Autodesk Inventor part; units mm, degrees
ref_plane "Work Plane1" through (0, -35, 0) normal (0, 1, 0) x (-1, 0, 0)
ref_plane "YZ Plane" through (0, 0, 0) normal (1, 0, 0) x (0, 1, 0)
ref_plane "XY Plane" through (0, 0, 0) normal (0, 0, 1) x (1, 0, 0)
sketch "Sketch1" plane through (0, 0, 0) normal (0, 0, 1) x (1, 0, 0)
  circle A0 centre (0, 0) radius 25
  circle A1 centre (0, 0) radius 35
  line L0 (-17.6777, 17.6777) -> (-24.7487, 24.7487)
  line L1 (0, 35) -> (0, 0) construction
  line L2 (-24.0315, 25.4457) -> (-16.9564, 18.3706)
  line L3 (-1.1667, 34.9806) -> (-1.1667, 34.9972)
  line L4 (1.1667, 34.9806) -> (1.1667, 34.9972)
  line L5 (17.6777, 17.6777) -> (24.7487, 24.7487)
  line L6 (24.0315, 25.4457) -> (16.9564, 18.3706)
  line L7 (-25.4457, 24.0315) -> (-18.3706, 16.9564)
  line L8 (25.4457, 24.0315) -> (18.3706, 16.9564)
  line L9 (-1, 15) -> (1, 15)
  line L10 (1, 15) -> (1, 0)
  line L11 (1, 0) -> (-1, 0)
  line L12 (-1, 0) -> (-1, 15)
  line L13 (-1, 0) -> (1, 0)
  line L14 (1, 0) -> (1, -7)
  line L15 (1, -7) -> (-1, -7)
  line L16 (-1, -7) -> (-1, 0)
  line L17 (-1, -7) -> (-5, -7)
  line L18 (-5, -7) -> (-5, 4)
  line L19 (-5, 4) -> (-1, 4)
  line L20 (-1, 4) -> (-1, -7)
  line L21 (-5, 4) -> (-21.5953, -12.5953)
  line L22 (-5, -7) -> (-16.6494, -18.6494)
  line L23 (-5, 4) -> (-1, 15)
  line L24 (-5, -7) -> (-1, -3)
  line L25 (1, 0) -> (1, 15)
  line L26 (1, -7) -> (1, 0)
  line L27 (5, 4) -> (21.5953, -12.5953)
  line L28 (5, -7) -> (16.6494, -18.6494)
  line L29 (5, 4) -> (1, 15)
  line L30 (5, -7) -> (1, -3)
  point P0 (-20.5061, 21.9203)
  point P1 (-21.9203, 20.5061)
  point P2 (20.5061, 21.9203)
  point P3 (21.9203, 20.5061)
  point P4 (-1, -3)
  point P5 (1, 0)
  point P6 (1, -3)
  point P7 (21.5953, -12.5953)
  dimension "d0" = 50
  dimension "d1" = 10
  dimension "d2" = 45
  dimension "d3" = 1
  dimension "d5" = 2
  dimension "d6" = 15
  dimension "d7" = 7
  dimension "d8" = 2
  dimension "d9" = 4
  dimension "d11" = 45
  dimension "d12" = 45
  dimension "d13" = 4
  dimension "d14" = 45
extrude "Extrusion1" add sketch "Sketch1" along normal blind 10 contours A0 L8 A1 L7 | A0 L28 L30 L14 L10 L29 L27 | A0 L21 L18 L22 | L18 L19 L12 L16 L24 | L12 L19 L23
sketch "Sketch2" plane through (0, 0, 0) normal (0, 0, 1) x (1, 0, 0)
  point P0 (0, 0)
extrude "Extrusion2" add sketch "Sketch1" along normal blind 5 contours A0 L5 A1 L8 | A0 L6 A1 L5 | A0 L2 A1 L6 | A0 L0 A1 L2 | A1 L0 A0 L7
sketch "Sketch4" plane through (0, 0, 5) normal (0, 0, 1) x (1, 0, 0)
  arc A0 (18.3706, 16.9564) -> (-18.3706, 16.9564) centre (0, 0) ccw construction
  circle A1 centre (0, 30) radius 2.5
  point P0 (0, 25)
  dimension "d19" = 5
  dimension "d20" = 5
extrude "Extrusion3" cut sketch "Sketch4" against normal through all
chamfer "Chamfer1" distance 1 angle 45 1 edges at (-2.5, 30, 5)
ref_plane "Work Plane1" through (0, -35, 0) normal (0, 1, 0) x (-1, 0, 0)
sketch "Sketch6" plane through (0, -35, 0) normal (0, 1, 0) x (-1, 0, 0)
  line L0 (3.5, 5) -> (-3.5, 5) construction
  circle A0 centre (0, 5) radius 4.9
  point P0 (0, 0)
  dimension "d27" = 9.8
extrude "Extrusion4" add sketch "Sketch6" along normal blind 5 and the other way blind 20
chamfer "Chamfer2" distance 1 angle 45 1 edges at (4.9, -55, 5)
properties part number "Black_Part1"
Verification items for the finished model (mm, model axes). A direction names the side the tool comes from. Round coordinates to 2 decimals unless told otherwise and drop trailing zeros. Order: outer loops, then holes, each group sorted by start corner. A loop starts at its lowest first (then second) coordinate and runs counter-clockwise, first axis right, second up. Notation, with made-up numbers: (9, 5.5) -> (68, 5.5) arc R23 ccw to (68, 13.5) -> close; hole circle Ø5 at (20.25, 45.25). An arc over 180 degrees is marked (long way). Put each result on its own line as item: value. Start each with the question number.
(1) Section check A-A (y = 0). Enter the section's corners in (x, z).
(2) Draft check along Y on faces 1 (the face through (3.03, 9.42, 4.93)), 2 (the face through (21.958, 20.543, 7.465)), 3 (the face through (0, 26, 5)). Enter one of: +Y half, -Y half, draft (parallel to the pull), parting line (faces both ways), or undercut.
(3) Material ranges on line 1 along Y through (x, z) = (0, 1.35); line 2 along Y through (x, z) = (9, 0.5); line 3 along X through (y, z) = (0, 3.5), recorded low to high.
(4) Section check D-D (y = -44.5). Enter the section's corners in (x, z), then the cut area to 3 significant figures.
(5) Section check B-B (y = 30). Enter the section's corners in (x, z), then the cut area to 3 significant figures.
(6) Depth check by flat-ended pin: pin 1 Ø6 at (y, z) = (-24, 8.5) entering from -X; pin 2 Ø1.5 at (y, z) = (-11, 9) entering from -X; pin 3 Ø1.5 at (x, z) = (26.5, 1.5) entering from -Y. Enter the tip coordinate at first touch or a pass-through.
(7) Section check C-C (x = -8.5). Enter the section's corners in (y, z).
(8) Tool access check on faces 4 (the face through (0, -25, 5)), 5 (the face through (-21.958, 20.543, 7.465)), 6 (the face through (0, -55, 5)), 7 (the face through (1.062, -44.463, 9.783)), 8 (the face through (7, 0, 0)). Record the directions out of +Z, -Z, +X, -X, +Y, -Y that give a thin tool (end or side, any length) a straight path to the whole face; none if there is none.
Completed:
1. outline: (-35, 0) -> (-25, 0) -> (-25, 10) -> (-35, 10) -> close; (-9, 0) -> (-1, 0) -> (-1, 10) -> (-9, 10) -> close; (1, 0) -> (9, 0) -> (9, 10) -> (1, 10) -> close; (25, 0) -> (35, 0) -> (35, 10) -> (25, 10) -> close
2. face 1: undercut
2. face 2: +Y half
2. face 3: draft
3. line 1: y = -55 to -25, 25 to 27.5, 32.5 to 35
3. line 2: y = -33.82 to -23.32, -11 to 0, 23.32 to 33.82
3. line 3: x = -35 to -25, -9 to -1, 1 to 9, 25 to 35
4. outline: circle Ø9.8 at (0, 5)
4. area: 75.4 mm2
5. outline: (-18.03, 0) -> (-2.5, 0) -> (-2.5, 4) -> (-3.5, 5) -> (-18.03, 5) -> close; (2.5, 0) -> (18.03, 0) -> (18.03, 5) -> (3.5, 5) -> (2.5, 4) -> close
5. area: 154 mm2
6. pin 1: stops at x = -28
6. pin 2: stops at x = -33.47
6. pin 3: stops at y = -23.71
7. outline: (-33.95, 0) -> (-23.51, 0) -> (-23.51, 10) -> (-33.95, 10) -> close; (-10.5, 0) -> (0.5, 0) -> (0.5, 10) -> (-10.5, 10) -> close; (23.51, 0) -> (33.95, 0) -> (33.95, 5) -> (23.51, 5) -> close
8. face 4: +Z, -Z
8. face 5: +Z, +Y
8. face 6: +Z, -Z, +X, -X, -Y
8. face 7: -Y
8. face 8: -Z, +X, -X, +Y, -Y
